from build123d import *

# Parameters (mm, degrees)
SKETCH2_W               = 60
SKETCH2_H               = 9.4666089
BOSS_EXTRUDE2_DEPTH     = 10
SKETCH3_W               = 10
SKETCH3_H               = 15
BOSS_EXTRUDE3_DEPTH     = 60
SKETCH4_W               = 10
SKETCH4_H               = 15
BOSS_EXTRUDE4_DEPTH     = 64.0502592
SKETCH6_R               = 9.5
SKETCH6_R_2             = 7.5
EXTRUDE_THIN1_DEPTH     = 10
CUT_EXTRUDE1_DEPTH      = 160.787854054
CUT_EXTRUDE1_DEPTH_BACK = 160.787854054
SKETCH8_W               = 15
SKETCH8_H               = 10
BOSS_EXTRUDE5_DEPTH     = 80
SKETCH9_R               = 2.95
BOSS_EXTRUDE6_DEPTH     = 150
SKETCH10_R              = 2.95
BOSS_EXTRUDE7_DEPTH     = 60


with BuildPart() as part:
    # Sketch2 → Boss-Extrude2 (new body)
    with BuildSketch(Plane(origin=(0, 0, 0), x_dir=(1, 0, 0), z_dir=(0, 1, 0))):
        Polygon((60, -15), (-60, -15), (-60, 0), (-45, 0), (-45, 9.4666089), (-60, 9.4666089), (-60, 24.4666089), (60, 24.4666089), (60, 9.4666089), (45, 9.4666089), (45, 0), (60, 0), align=None)
        with Locations((0, 4.73330445)):
            Rectangle(SKETCH2_W, SKETCH2_H, mode=Mode.SUBTRACT)
    extrude(amount=BOSS_EXTRUDE2_DEPTH)

    # Sketch3 → Boss-Extrude3 (add)
    with BuildSketch(Plane(origin=(0, 10, 0), x_dir=(1, 0, 0), z_dir=(0, 1, 0))):
        with Locations((0, -7.5)):
            Rectangle(SKETCH3_W, SKETCH3_H)
        with Locations((0, 16.9666089)):
            Rectangle(SKETCH3_W, SKETCH3_H)
    extrude(amount=BOSS_EXTRUDE3_DEPTH)

    # Sketch4 → Boss-Extrude4 (add)
    with BuildSketch(Plane(origin=(0, 70, 0), x_dir=(1, 0, 0), z_dir=(0, 1, 0))):
        with Locations((0, 16.9666089)):
            Rectangle(SKETCH4_W, SKETCH4_H)
    extrude(amount=BOSS_EXTRUDE4_DEPTH)

    # Sketch6 → Extrude-Thin1 (add, symmetric)
    # profile 1 of 2: a face of its own
    with BuildSketch(Plane(origin=(0, 0, 0), x_dir=(0, 0, -1), z_dir=(1, 0, 0))):
        with Locations((-7.5, 70)):
            Circle(SKETCH6_R)
        with Locations((-7.5, 70)):
            Circle(SKETCH6_R_2, mode=Mode.SUBTRACT)
    # profile 2 of 2: a face of its own
    with BuildSketch(Plane(origin=(0, 0, 0), x_dir=(0, 0, -1), z_dir=(1, 0, 0))):
        with Locations((16.9666089, 134.0502592)):
            Circle(SKETCH6_R)
        with Locations((16.9666089, 134.0502592)):
            Circle(SKETCH6_R_2, mode=Mode.SUBTRACT)
    extrude(amount=EXTRUDE_THIN1_DEPTH, both=True)

    # Sketch7 → Cut-Extrude1 (cut, two sides: drawn at the far end of the back side and taken through both)
    with BuildSketch(Plane(origin=(5, 0, 0), x_dir=(0, 0, -1), z_dir=(1, 0, 0)).offset(-CUT_EXTRUDE1_DEPTH_BACK)):
        with BuildLine():
            Line((0, 70), (-15, 70))
            ThreePointArc((-15, 70), (-7.5, 62.5), (0, 70))
        make_face()
        with BuildLine():
            Line((24.4666089, 134.0502592), (9.4666089, 134.0502592))
            ThreePointArc((9.4666089, 134.0502592), (16.9666089, 126.5502592), (24.4666089, 134.0502592))
        make_face()
    extrude(amount=CUT_EXTRUDE1_DEPTH + CUT_EXTRUDE1_DEPTH_BACK, mode=Mode.SUBTRACT)

    # Sketch8 → Boss-Extrude5 (add)
    with BuildSketch(Plane.XZ):
        with Locations((37.5, -4.75)):
            Rectangle(SKETCH8_W, SKETCH8_H)
    extrude(amount=BOSS_EXTRUDE5_DEPTH)

    # Sketch9 → Boss-Extrude6 (add)
    with BuildSketch(Plane.ZY.offset(-30)):
        with Locations((-4.75, -75)):
            Circle(SKETCH9_R)
    extrude(amount=BOSS_EXTRUDE6_DEPTH)

    # Sketch10 → Boss-Extrude7 (add)
    with BuildSketch(Plane.ZY.offset(60)):
        with Locations(Location((7.5, 5, 0), (0, 0, 180))):
            Circle(SKETCH10_R)
    extrude(amount=BOSS_EXTRUDE7_DEPTH)


solid = part.part
Verification items for the finished model (mm, model axes). A direction names the side the tool comes from. Round coordinates to 2 decimals unless told otherwise and drop trailing zeros. Loops run counter-clockwise (first coordinate to the right, second up) from the corner with the lowest first, then second, coordinate; pieces in that order, holes last. Notation, with made-up numbers: (54.25, -1.5) - (83.25, -1.5) arc R10 ccw to (83.25, 10.5) - close; hole circle Ø3 at (72, 61.25). An arc over 180 degrees is marked (long way). Use a Markdown table: item, result. Add a question column.
1. Thickness scan on probe 1 along X at (y, z) = (56, -24); probe 2 along Y at (x, z) = (38, -3); probe 3 along Y at (x, z) = (-28, -18). Record the ranges inside material, lowest first. Write a range as [from, to].
2. Gauge pin test, flat ends, axial feed: pin 1 (19.5 mm diameter, centred on x = -22.5, y = 27.5, fed in from +Z); pin 2 (8 mm diameter, centred on y = -23, z = -3.5, fed in from +X); pin 3 (4 mm diameter, centred on y = -46.5, z = -7.5, fed in from -X); pin 4 (17 mm diameter, centred on y = 134.05, z = -16.97, fed in from -X). Record the tip position at first contact, or that the pin passes through.
3. Section check B-B, the plane z = -4.75. Record the boundary of the cut face in (x, y).
4. Release check for a two-part mould opening along Y. For faces 1 (the face through (5, 37, 8)), 2 (the face through (-2, 20, 0)), 3 (the face through (37, -80, -5)) record: released by +Y, released by -Y, zero draft, split by the parting line, or undercut.
5. Section check D-D, the plane y = 35. Record the boundary of the cut face in (x, z).
6. Section check A-A, the plane x = -15.5. Record the boundary of the cut face in (y, z).
7. Access from +Z, -Z, +X, -X, +Y, -Y to the whole of each face (thin tool, end or side, straight path). Record for faces 4 (the face through (-60, 5, -17)), 5 (the face through (0, 50, -9.467)), 6 (the face through (52, 5, 0)), 7 (the face through (37, -39, -9.75)), 8 (the face through (0, 18, 15)).
8. Section check C-C, the plane y = 5. Record the boundary of the cut face in (x, z).
Checks:
| question | item | result |
|---|---|---|
| 1 | probe 1 | x = [-5, 5] |
| 1 | probe 2 | y = [-80, 10] |
| 1 | probe 3 | y = [0, 10] |
| 2 | pin 1 | passes through |
| 2 | pin 2 | stops at x = 45 |
| 2 | pin 3 | stops at x = 30 |
| 2 | pin 4 | stops at x = -10 |
| 3 | outline | (-120, -77.95) - (30, -77.95) - (30, -80) - (45, -80) - (45, 10) - (30, 10) - (30, -72.05) - (-120, -72.05) - close; (-45, 0) - (-30, 0) - (-30, 10) - (-45, 10) - close |
| 4 | face 1 | undercut |
| 4 | face 2 | zero draft |
| 4 | face 3 | released by -Y |
| 5 | outline | (-5, -24.47) - (5, -24.47) - (5, -9.47) - (-5, -9.47) - close; (-5, 0) - (5, 0) - (5, 15) - (-5, 15) - close |
| 6 | outline | circle Ø5.9 at (-75, -4.75); (0, -24.47) - (10, -24.47) - (10, -9.47) - (0, -9.47) - close; (0, 0) - (10, 0) - (10, 15) - (0, 15) - close |
| 7 | face 4 | -Z, -X, +Y, -Y |
| 7 | face 5 | -Y |
| 7 | face 6 | +X, +Y, -Y |
| 7 | face 7 | -Z, +X, -X, -Y |
| 7 | face 8 | +Z, +X, -X, -Y |
| 8 | outline | (-120, 4.55) - (-60, 4.55) - (-60, 0) - (-45, 0) - (-45, -9.47) - (-60, -9.47) - (-60, -24.47) - (60, -24.47) - (60, -9.47) - (45, -9.47) - (45, 0) - (60, 0) - (60, 15) - (-60, 15) - (-60, 10.45) - (-120, 10.45) - close; hole (-30, -9.47) - (30, -9.47) - (30, 0) - (-30, 0) - close |
